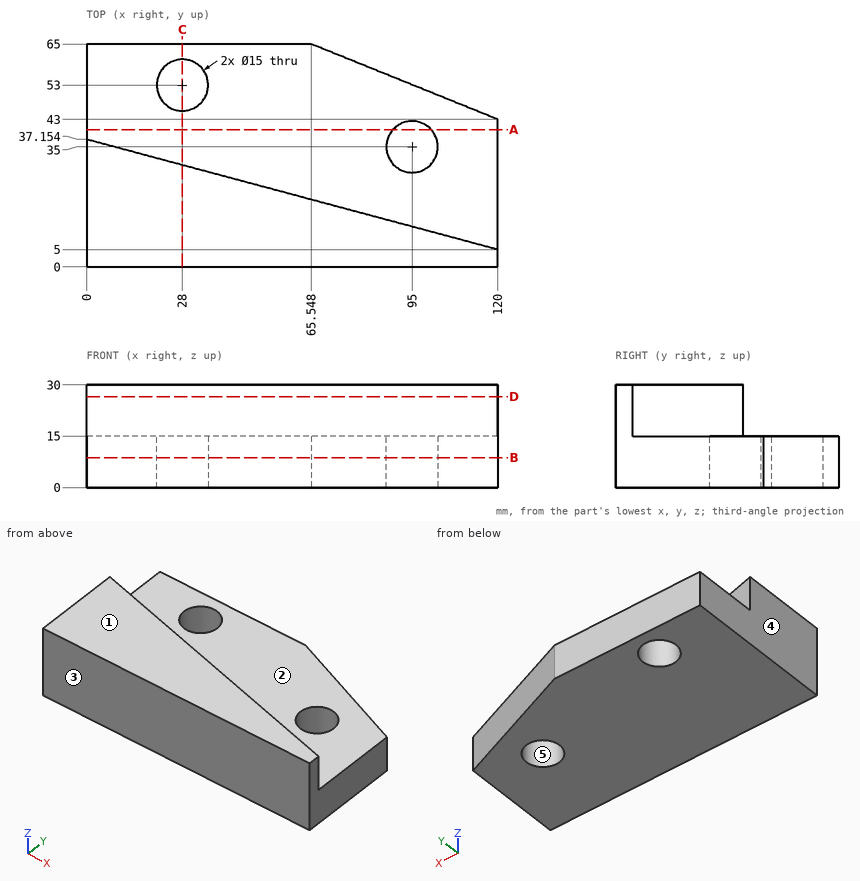
Design review of the part shown in the three views and the two pictorial views. Dimensions are in mm from the part's minimum x, y and z. A direction names the side the tool comes from. Round coordinates to 2 decimals unless told otherwise and drop trailing zeros. Write each loop counter-clockwise with the first axis right and the second up, starting at its lowest first coordinate (ties: lowest second). Pieces come first, ordered by that corner, then holes.
1) Machinability: for the marked faces 1 and 2, which of the approach directions +Z, -Z, +X, -X, +Y, -Y give a long, thin tool a straight path to every point of the face, cutting with its end or side? Answer none if there is none.
Answer below:
face 1: +Z, +X, -X, +Y, -Y
face 2: +Z, +X, +Y
2) Take a section at C-C on x = 28. Give the boundary of the cut face in (y, z), then the cut area to 3 significant figures.
Answer below:
outline: (0, 0) - (45.5, 0) - (45.5, 15) - (29.65, 15) - (29.65, 30) - (0, 30) - close; (60.5, 0) - (65, 0) - (65, 15) - (60.5, 15) - close
area: 1,190 mm2
3) Take a section at B-B on z = 8.75. Give the boundary of the cut face in (x, y), then the cut area to 3 significant figures.
Answer below:
outline: (0, 0) - (120, 0) - (120, 43) - (65.55, 65) - (0, 65) - close; hole circle Ø15 at (28, 53); hole circle Ø15 at (95, 35)
area: 6,850 mm2
4) Take a section at A-A on y = 40. Give the boundary of the cut face in (x, z).
Answer below:
outline: (0, 0) - (89.41, 0) - (89.41, 15) - (0, 15) - close; (100.59, 0) - (120, 0) - (120, 15) - (100.59, 15) - close
5) For line 1 along Y through (x, z) = (28, 9.75); line 2 along Z through (x, y) = (16, 36.5); line 3 along Y through (x, z) = (95, 10.75), list the stretches that pass through material, from the lowest coordinate up.
Answer below:
line 1: y = 0 to 45.5, 60.5 to 65
line 2: z = 0 to 15
line 3: y = 0 to 27.5, 42.5 to 53.1
6) Mouldability with a two-part tool opening along Y and no side actions: class the marked faces 3, 4 and 5 as +Y half, -Y half, draft (parallel to the pull), parting line (faces both ways), or undercut.
Answer below:
face 3: -Y half
face 4: draft
face 5: undercut
7) Insertion check: pin 1 Ø1.5 at (y, z) = (54, 12.5) entering from +X; pin 2 Ø3 at (y, z) = (12.5, 13.5) entering from -X; pin 3 Ø1 at (x, y) = (49.5, 25) entering from +Z; pin 4 Ø9 at (x, y) = (28, 53) entering from -Z. Each pin has a flat end and moves straight along its axis. Give the tip position at first contact, or say it passes through.
Answer below:
pin 1: stops at x = 94.63
pin 2: stops at x = 0
pin 3: stops at z = 15
pin 4: passes through
8) Take a section at D-D on z = 26.5. Give the boundary of the cut face in (x, y).
Answer below:
outline: (0, 0) - (120, 0) - (120, 5) - (0, 37.15) - close
